from build123d import *

# Parameters (mm, degrees)
PAD_DEPTH       = 80
SKETCH001_R     = 1.65
POCKET_DEPTH    = 13.501
SKETCH002_R     = 3
POCKET001_DEPTH = 6
SKETCH003_R     = 10.65
POCKET002_DEPTH = 30.4
SKETCH004_R     = 10.65
POCKET003_DEPTH = 30.4
FILLET_R        = 5


with BuildPart() as part:
    # Sketch → Pad (new body)
    with BuildSketch(Plane.XZ):
        with BuildLine():
            Line((20, 0), (20, -13.5))
            Line((20, -13.5), (-20, -13.5))
            Line((-20, -13.5), (-20, 0))
            Line((-20, 0), (-7, 0))
            ThreePointArc((-7, 0), (0, -7), (7, 0))
            Line((7, 0), (20, 0))
        make_face()
    extrude(amount=PAD_DEPTH)

    # Sketch001 → Pocket (cut, through all)
    with BuildSketch(Plane.XY):
        with Locations((-15, -5)):
            Circle(SKETCH001_R)
        with Locations((-15, -40)):
            Circle(SKETCH001_R)
        with Locations((-15, -75)):
            Circle(SKETCH001_R)
        with Locations((15, -5)):
            Circle(SKETCH001_R)
        with Locations((15, -40)):
            Circle(SKETCH001_R)
        with Locations((15, -75)):
            Circle(SKETCH001_R)
    extrude(amount=-POCKET_DEPTH, mode=Mode.SUBTRACT)

    # Sketch002 (on DatumPlane) → Pocket001 (cut)
    with BuildSketch(Plane.XY.offset(-13.5)):
        with Locations((-15, -5)):
            Circle(SKETCH002_R)
        with Locations((-15, -40)):
            Circle(SKETCH002_R)
        with Locations((-15, -75)):
            Circle(SKETCH002_R)
        with Locations((15, -5)):
            Circle(SKETCH002_R)
        with Locations((15, -40)):
            Circle(SKETCH002_R)
        with Locations((15, -75)):
            Circle(SKETCH002_R)
    extrude(amount=POCKET001_DEPTH, mode=Mode.SUBTRACT)

    # Sketch003 (on DatumPlane) → Pocket002 (cut)
    with BuildSketch(Plane.XZ.offset(5)):
        Circle(SKETCH003_R)
    extrude(amount=POCKET002_DEPTH, mode=Mode.SUBTRACT)

    # Sketch004 (on DatumPlane) → Pocket003 (cut)
    with BuildSketch(Plane.XZ.offset(75)):
        Circle(SKETCH004_R)
    extrude(amount=-POCKET003_DEPTH, mode=Mode.SUBTRACT)

    # Fillet
    fillet_edges = [part.edges().sort_by_distance(p)[0] for p in [
        (-20, -80, -6.75),
    ]]
    fillet(fillet_edges, radius=FILLET_R)


solid = part.part
Geometry: final body of the model. Coordinates: model frame, mm. A direction names the side the tool comes from. Coordinates: 2 decimals unless noted, no trailing zeros. Order: outer loops, then holes, each group sorted by start corner. A loop starts at its lowest first (then second) coordinate and runs counter-clockwise, first axis right, second up.
1) Section C-C (z = -0.75). Give the number of separate pieces and of enclosed holes in the cut face, then the cut area to 3 significant figures.
Result sheet:
separate pieces: 2
enclosed holes: 6
area: 1,580 mm2
2) Ray query, probe 1 along Y at (x, z) = (-15, -9.05); probe 2 along Y at (x, z) = (-15, -2.75); probe 3 along Y at (x, z) = (8, -6). Return the intervals inside material, ascending.
Result sheet:
probe 1: y = -80 to -78, -72 to -43, -37 to -8, -2 to 0
probe 2: y = -80 to -76.65, -73.35 to -41.65, -38.35 to -6.65, -3.35 to 0
probe 3: y = -80 to -75, -44.6 to -35.4, -5 to 0
3) Section D-D (z = -12). Return loops of the section in (x, y).
Result sheet:
outline: (-20, -75) arc R5 ccw to (-15, -80) - (20, -80) - (20, 0) - (-20, 0) - close; hole circle Ø6 at (-15, -75); hole circle Ø6 at (-15, -40); hole circle Ø6 at (-15, -5); hole circle Ø6 at (15, -75); hole circle Ø6 at (15, -40); hole circle Ø6 at (15, -5)
4) First-contact query: P1, Ø1.8, axis at x = -16, y = -39, coming from the -Z side. Flat tip, straight axial feed; report the tip coordinate or a pass-through.
Result sheet:
P1: stops at z = -7.5
5) Section B-B (y = -40). Return loops of the section in (x, z).
Result sheet:
outline: (-20, -13.5) - (-18, -13.5) - (-18, -7.5) - (-16.65, -7.5) - (-16.65, 0) - (-20, 0) - close; (-13.35, -7.5) - (-12, -7.5) - (-12, -13.5) - (12, -13.5) - (12, -7.5) - (13.35, -7.5) - (13.35, 0) - (7, 0) arc R7 cw to (-7, 0) - (-13.35, 0) - close; (16.65, -7.5) - (18, -7.5) - (18, -13.5) - (20, -13.5) - (20, 0) - (16.65, 0) - close
6) Draft query along X for faces 4 (the flat face through (-12, -39, 0)), 5 (the cylindrical face through (-17.21, -2.97, -10.54)), 6 (the flat face through (20, -39, -7)). Return one class per face: released by +X, released by -X, zero draft, split by the parting line, or undercut.
Result sheet:
face 4: zero draft
face 5: undercut
face 6: released by +X
7) Set-up query: faces 1 (the flat face through (-13.7, -41.3, -7.5)), 2 (the flat face through (0, -44.6, -8)), 3 (the cylindrical face through (-13.476, -5.632, -3.698)). Return all of +Z, -Z, +X, -X, +Y, -Y with unobstructed straight access to the full face (end or side cutting, diameter ignored); none if empty.
Result sheet:
face 1: -Z
face 2: +Z
face 3: +Z, -Z
8) Section A-A (x = 15). Return loops of the section in (y, z).
Result sheet:
outline: (-80, -13.5) - (-78, -13.5) - (-78, -7.5) - (-76.65, -7.5) - (-76.65, 0) - (-80, 0) - close; (-73.35, -7.5) - (-72, -7.5) - (-72, -13.5) - (-43, -13.5) - (-43, -7.5) - (-41.65, -7.5) - (-41.65, 0) - (-73.35, 0) - close; (-38.35, -7.5) - (-37, -7.5) - (-37, -13.5) - (-8, -13.5) - (-8, -7.5) - (-6.65, -7.5) - (-6.65, 0) - (-38.35, 0) - close; (-3.35, -7.5) - (-2, -7.5) - (-2, -13.5) - (0, -13.5) - (0, 0) - (-3.35, 0) - close
